Input: part model. Units: mm. Frame: model coordinates. A direction names the side the tool comes from. Give positions to 0.01 mm unless a question says otherwise; leave off trailing zeros. Loops run counter-clockwise (first coordinate to the right, second up) from the corner with the lowest first, then second, coordinate; pieces in that order, holes last. Notation, with made-up numbers: (1, 80.25) -> (47, 80.25) arc R18 ccw to (47, 89.25) -> close; hole circle Ø7 at (9, 4.5). An arc over 180 degrees is marked (long way). Answer as a JSON object with one key per item and string values.
```python
from build123d import *

# Parameters (mm, degrees)
SKETCH1_R           = 2.5
BOSS_EXTRUDE1_DEPTH = 3
SKETCH2_W           = 5
SKETCH2_H           = 1
BOSS_EXTRUDE2_DEPTH = 3
SKETCH3_W           = 1
SKETCH3_H           = 3
BOSS_EXTRUDE3_DEPTH = 3


with BuildPart() as part:
    # Sketch1 → Boss-Extrude1 (new body)
    with BuildSketch(Plane.XY):
        Polygon((0, 10), (10, 7.132546142), (10, 2.5), (5, 2.5), (5, -2.5), (10, -2.5), (10, -7.132546142), (0, -10), (-10, -10), (-10, 10), align=None)
        with Locations((-5, 0)):
            Circle(SKETCH1_R, mode=Mode.SUBTRACT)
    extrude(amount=BOSS_EXTRUDE1_DEPTH)

    # Sketch2 → Boss-Extrude2 (add)
    with BuildSketch(Plane(origin=(0, 0, 0), x_dir=(-1, 0, 0), z_dir=(0, 0, -1))):
        with Locations((-7.5, 2)):
            Rectangle(SKETCH2_W, SKETCH2_H)
        with Locations((-7.5, -2)):
            Rectangle(SKETCH2_W, SKETCH2_H)
    extrude(amount=-BOSS_EXTRUDE2_DEPTH)

    # Sketch3 → Boss-Extrude3 (add)
    with BuildSketch(Plane(origin=(0, 0, 0), x_dir=(-1, 0, 0), z_dir=(0, 0, -1))):
        with Locations((-5.5, 0)):
            Rectangle(SKETCH3_W, SKETCH3_H)
    extrude(amount=-BOSS_EXTRUDE3_DEPTH)


solid = part.part
```
Q1. Draft query along Y for faces 3 (the flat face through (10, -4, 1)), 4 (the flat face through (-5, 10, 1)), 5 (the flat face through (8, 1.5, 1)). Return one class per face: +Y half, -Y half, draft (parallel to the pull), parting line (faces both ways), or undercut.
Evaluation:
{"face 3": "draft", "face 4": "+Y half", "face 5": "undercut"}
Q2. Pin query (flat end, axial travel): pin 1 (0.9 mm diameter, centred on x = 8, z = 2, fed in from -Y); pin 2 (1.5 mm diameter, centred on y = -0.5, z = 2, fed in from +X); pin 3 (1.5 mm diameter, centred on x = 8.5, z = 1.5, fed in from +Y); pin 4 (3 mm diameter, centred on x = -5, y = 0, fed in from +Z). Return the tip coordinate at first contact, or that it passes through.
Evaluation:
{"pin 1": "stops at y = -7.84", "pin 2": "stops at x = 6", "pin 3": "stops at y = 7.78", "pin 4": "passes through"}
Q3. Section A-A, the plane x = -5. Return the cut outline in (y, z).
Evaluation:
{"outline": "(-10, 0) -> (-2.5, 0) -> (-2.5, 3) -> (-10, 3) -> close; (2.5, 0) -> (10, 0) -> (10, 3) -> (2.5, 3) -> close"}
Q4. Section C-C, the plane z = 0.6. Return the cut outline in (x, y).
Evaluation:
{"outline": "(-10, -10) -> (0, -10) -> (10, -7.13) -> (10, -1.5) -> (6, -1.5) -> (6, 1.5) -> (10, 1.5) -> (10, 7.13) -> (0, 10) -> (-10, 10) -> close; hole circle Ø5 at (-5, 0)"}
Q5. Ray query, line 1 along Y through (x, z) = (-5, 1.1); line 2 along Y through (x, z) = (7.25, 1.3); line 3 along X through (y, z) = (2.25, 1.15). Return the intervals inside material, ascending.
Evaluation:
{"line 1": "y = -10 to -2.5, 2.5 to 10", "line 2": "y = -7.92 to -1.5, 1.5 to 7.92", "line 3": "x = -10 to -6.09, -3.91 to 10"}
Q6. Section B-B, the plane y = 0. Return the cut outline in (x, z), then the cut area to 3 significant figures.
Evaluation:
{"outline": "(-10, 0) -> (-7.5, 0) -> (-7.5, 3) -> (-10, 3) -> close; (-2.5, 0) -> (6, 0) -> (6, 3) -> (-2.5, 3) -> close", "area": "33.0 mm2"}
Q7. Access query for faces 1 (the flat face through (0, 0, 3)), 2 (the flat face through (8, -1.5, 1)). Directions: +Z, -Z, +X, -X, +Y, -Y. A direction counts if a zero-diameter tool reaches every point of the face in a straight line with its end or side. Return the directions, or none.
Evaluation:
{"face 1": "+Z, +X, -X, +Y, -Y", "face 2": "+Z, -Z, +X"}
